from build123d import *

# Parameters (mm, degrees)
BOSS_EXTRUDE1_DEPTH = 9
SKETCH2_R           = 1.55
CUT_EXTRUDE1_DEPTH  = 19


with BuildPart() as part:
    # Sketch1 → Boss-Extrude1 (new body)
    with BuildSketch(Plane(origin=(0, 0, 0), x_dir=(1, 0, 0), z_dir=(0, 1, 0))):
        with BuildLine():
            Line((12.15, 0), (26.4, 0))
            Line((26.4, 0), (26.4, 18))
            Line((26.4, 18), (-26.4, 18))
            Line((-26.4, 18), (-26.4, 0))
            Line((-26.4, 0), (-12.15, 0))
            ThreePointArc((-12.15, 0), (0, 12.15), (12.15, 0))
        make_face()
    extrude(amount=BOSS_EXTRUDE1_DEPTH)

    # Sketch2 → Cut-Extrude1 (cut, through all)
    with BuildSketch(Plane.XY):
        with Locations((21.4, 4.5)):
            Circle(SKETCH2_R)
    cut_extrude1 = extrude(amount=-CUT_EXTRUDE1_DEPTH, mode=Mode.SUBTRACT)

    # Mirror1: Cut-Extrude1 across plane
    add(cut_extrude1.mirror(Plane(origin=(0, 0, 0), x_dir=(0, 0, 1), z_dir=(1, 0, 0))), mode=Mode.SUBTRACT)


solid = part.part
CAD build for the part. Positions are in the model's coordinates, mm. Coordinates: 2 decimals unless noted, no trailing zeros. Order: outer loops, then holes, each group sorted by start corner. A loop starts at its lowest first (then second) coordinate and runs counter-clockwise, first axis right, second up.
Item 1: Band-saw the part on D-D on z = -1. List the corners of the cut face in (x, y), plus the area to 3 significant figures.
Check sheet entries:
outline: (-26.4, 0) - (-12.11, 0) - (-12.11, 9) - (-26.4, 9) - close; (12.11, 0) - (26.4, 0) - (26.4, 9) - (12.11, 9) - close; hole circle Ø3.1 at (-21.4, 4.5); hole circle Ø3.1 at (21.4, 4.5)
area: 242 mm2
Item 2: Band-saw the part on A-A on x = 21.4. List the corners of the cut face in (y, z), plus the area to 3 significant figures.
Check sheet entries:
outline: (0, -18) - (2.95, -18) - (2.95, 0) - (0, 0) - close; (6.05, -18) - (9, -18) - (9, 0) - (6.05, 0) - close
area: 106 mm2
Item 3: Two-plate mould, pull along X, no slides. Class faces 1 (the face through (-22.832, 3.906, -8.874)), 2 (the face through (19, 4, 0)), 3 (the face through (-26.4, 4, -9)): +X half, -X half, draft (parallel to the pull), parting line (faces both ways), or undercut.
Check sheet entries:
face 1: undercut
face 2: draft
face 3: -X half
Item 4: Pin check, flat tips, straight feed: pin 1 Ø3 at (x, y) = (-21.4, 4.5) entering from +Z; pin 2 Ø4 at (x, z) = (-8, -14) entering from -Y. Stop position of each tip, or through.
Check sheet entries:
pin 1: passes through
pin 2: stops at y = 0
Item 5: Band-saw the part on C-C on y = 4.5. List the corners of the cut face in (x, z).
Check sheet entries:
outline: (-26.4, -18) - (-22.95, -18) - (-22.95, 0) - (-26.4, 0) - close; (-19.85, -18) - (19.85, -18) - (19.85, 0) - (12.15, 0) arc R12.15 cw to (-12.15, 0) - (-19.85, 0) - close; (22.95, -18) - (26.4, -18) - (26.4, 0) - (22.95, 0) - close
Item 6: Drill centre lines: L1, parallel to Y at x = -21.4, z = -13; L2, parallel to X at y = 5.75, z = -14; L3, parallel to X at y = 1.5, z = -10. Where is each one in solid material? Low to high.
Check sheet entries:
L1: y = 0 to 2.95, 6.05 to 9
L2: x = -26.4 to -22.32, -20.48 to 20.48, 22.32 to 26.4
L3: x = -26.4 to -6.9, 6.9 to 26.4
Item 7: Band-saw the part on B-B on z = -7.25. List the corners of the cut face in (x, y).
Check sheet entries:
outline: (-26.4, 0) - (-9.75, 0) - (-9.75, 9) - (-26.4, 9) - close; (9.75, 0) - (26.4, 0) - (26.4, 9) - (9.75, 9) - close; hole circle Ø3.1 at (-21.4, 4.5); hole circle Ø3.1 at (21.4, 4.5)
